Can you work these out from the drawing? Everything is in mm from the part's minimum corner. A direction names the side the tool comes from. Coordinates: 2 decimals unless noted, no trailing zeros. Order: outer loops, then holes, each group sorted by start corner. A loop starts at its lowest first (then second) coordinate and runs counter-clockwise, first axis right, second up. Notation, with made-up numbers: (-14.5, 44.5) - (-9.5, 44.5) arc R27 ccw to (-9.5, 63.5) - close; hole circle Ø9 at (-5.5, 25). An arc over 180 degrees is marked (long way). Answer as CSV lines item,"result". Start each with the question number.
Item 1: Imagine slicing it at D-D on z = 33.5. List the corners of the cut face in (x, y) for me, and give its area (3 significant figures).
Item 2: We'd pull the mould along Z, two halves only. Please class the marked faces 5, 6 and 7: pulls with the +Z half, pulls with the -Z half, needs draft (parallel to the pull), parting line crosses it, or undercut.
Item 3: Imagine slicing it at B-B on x = 10. List the corners of the cut face in (y, z) for me, and give its area (3 significant figures).
Item 4: I need wall thicknesses on line 1 (Y direction, x = 65.5, z = 30); line 2 (Z direction, x = 59.5, y = 15); line 3 (X direction, y = 24.25, z = 2). Which ranges of each line are inside material? Lowest first, please.
Item 5: I'm going to push flat-ended pins straight in: pin 1 (4 mm diameter, centred on x = 30, y = 18, fed in from -Z); pin 2 (15 mm diameter, centred on x = 32, y = 19, fed in from +Z); pin 3 (5 mm diameter, centred on y = 3.5, z = 15.5, fed in from -X). Where does each tip first touch, or does it pass through?
Item 6: Imagine slicing it at C-C on z = 10. List the corners of the cut face in (x, y) for me, and give its area (3 significant figures).
Item 7: On a 3-axis mill with a long thin cutter (end or side, diameter ignored), from which of +Z, -Z, +X, -X, +Y, -Y can I reach the whole of each face in a straight line? I mean the marked faces 1, 2, 3 and 4. Say none if no direction works.
Item 8: Imagine slicing it at A-A on y = 15. List the corners of the cut face in (x, z) for me.
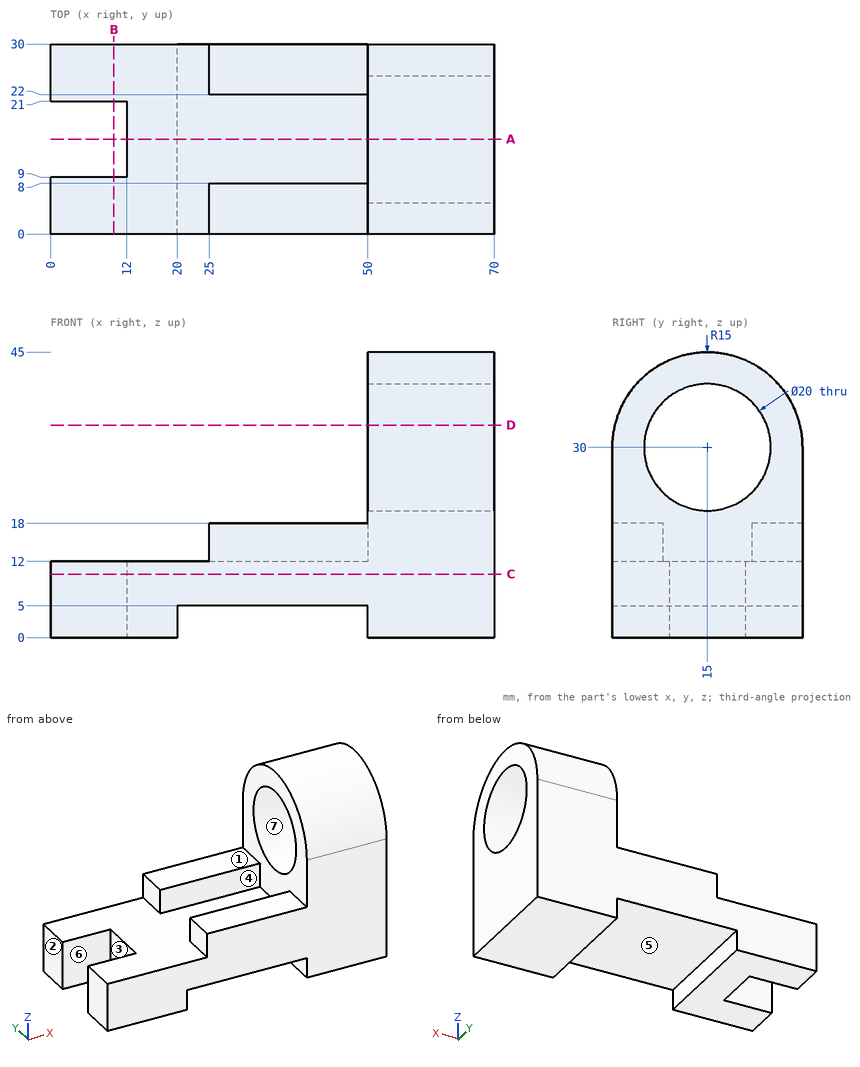
Responses:
1,outline,"(50, 0.41) - (70, 0.41) - (70, 5.63) - (50, 5.63) - close; (50, 24.37) - (70, 24.37) - (70, 29.59) - (50, 29.59) - close"
1,area,"209 mm^2"
2,face 5,"pulls with the -Z half"
2,face 6,"needs draft"
2,face 7,"undercut"
3,outline,"(0, 0) - (9, 0) - (9, 12) - (0, 12) - close; (21, 0) - (30, 0) - (30, 12) - (21, 12) - close"
3,area,"216 mm^2"
4,line 1,"y = 0 to 5, 25 to 30"
4,line 2,"z = 0 to 20, 40 to 45"
4,line 3,"x = 0 to 20, 50 to 70"
5,pin 1,"stops at z = 5"
5,pin 2,"stops at z = 18"
5,pin 3,"stops at x = 25"
6,outline,"(0, 0) - (70, 0) - (70, 30) - (0, 30) - (0, 21) - (12, 21) - (12, 9) - (0, 9) - close"
6,area,"1,960 mm^2"
7,face 1,"+Z, -X, +Y, -Y"
7,face 2,"+Z, -Z, -X, +Y, -Y"
7,face 3,"+Z, -Z, -X"
7,face 4,"+Z, -X"
8,outline,"(12, 0) - (20, 0) - (20, 5) - (50, 5) - (50, 0) - (70, 0) - (70, 20) - (50, 20) - (50, 12) - (12, 12) - close; (50, 40) - (70, 40) - (70, 45) - (50, 45) - close"
